```python
from build123d import *

# Parameters (mm, degrees)
SKETCH1_R           = 29.25
SKETCH1_R_2         = 22.025
BOSS_EXTRUDE1_DEPTH = 7
CUT_EXTRUDE1_START  = 7
SKETCH1_3_R         = 1.55
CUT_EXTRUDE1_DEPTH  = 4
SKETCH4_R           = 22.25
SKETCH4_R_2         = 21
BOSS_EXTRUDE2_DEPTH = 1
SKETCH3_R           = 1.55
CUT_EXTRUDE2_DEPTH  = 42.953843686


with BuildPart() as part:
    # Sketch1 → Boss-Extrude1 (new body)
    with BuildSketch(Plane.XY):
        Circle(SKETCH1_R)
        Circle(SKETCH1_R_2, mode=Mode.SUBTRACT)
    extrude(amount=BOSS_EXTRUDE1_DEPTH)

    # Sketch1<3> → Cut-Extrude1 (cut)
    with BuildSketch(Plane.XY.offset(CUT_EXTRUDE1_START)):
        with Locations((0, 25)):
            Circle(SKETCH1_3_R)
        with Locations((10.847093478, 22.524221698)):
            Circle(SKETCH1_3_R)
        with Locations((19.545787062, 15.587245046)):
            Circle(SKETCH1_3_R)
        with Locations((24.373197805, 5.563023349)):
            Circle(SKETCH1_3_R)
        with Locations((24.373197805, -5.563023349)):
            Circle(SKETCH1_3_R)
        with Locations((19.545787062, -15.587245046)):
            Circle(SKETCH1_3_R)
        with Locations((10.847093478, -22.524221698)):
            Circle(SKETCH1_3_R)
        with Locations((0, -25)):
            Circle(SKETCH1_3_R)
        with Locations((-10.847093478, -22.524221698)):
            Circle(SKETCH1_3_R)
        with Locations((-19.545787062, -15.587245046)):
            Circle(SKETCH1_3_R)
        with Locations((-24.373197805, -5.563023349)):
            Circle(SKETCH1_3_R)
        with Locations((-24.373197805, 5.563023349)):
            Circle(SKETCH1_3_R)
        with Locations((-19.545787062, 15.587245046)):
            Circle(SKETCH1_3_R)
        with Locations((-10.847093478, 22.524221698)):
            Circle(SKETCH1_3_R)
    extrude(amount=-CUT_EXTRUDE1_DEPTH, mode=Mode.SUBTRACT)

    # Sketch4 → Boss-Extrude2 (add)
    with BuildSketch(Plane.XY):
        Circle(SKETCH4_R)
        Circle(SKETCH4_R_2, mode=Mode.SUBTRACT)
    extrude(amount=BOSS_EXTRUDE2_DEPTH)

    # Sketch3 → Cut-Extrude2 (cut, through all)
    with BuildSketch(Plane.XY):
        with Locations((5.89680475, 25.835589673)):
            Circle(SKETCH3_R)
        with Locations((23.875674999, 11.497919087)):
            Circle(SKETCH3_R)
        with Locations((23.875674999, -11.497919087)):
            Circle(SKETCH3_R)
        with Locations((5.89680475, -25.835589673)):
            Circle(SKETCH3_R)
        with Locations((-16.522479749, -20.718534285)):
            Circle(SKETCH3_R)
        with Locations((-26.5, 0)):
            Circle(SKETCH3_R)
        with Locations((-16.522479749, 20.718534285)):
            Circle(SKETCH3_R)
    extrude(amount=CUT_EXTRUDE2_DEPTH, mode=Mode.SUBTRACT)


solid = part.part
```
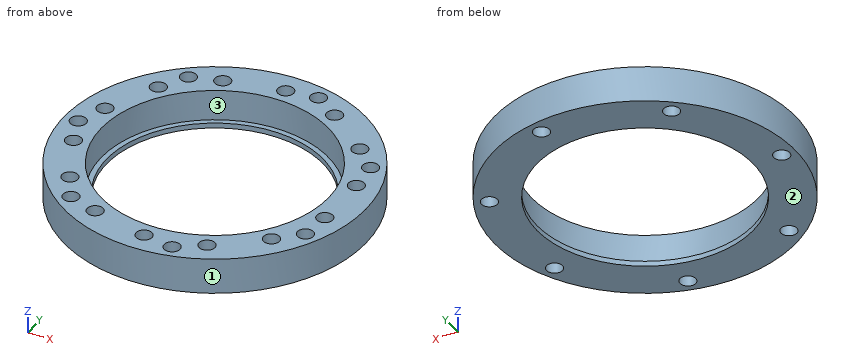
Geometry check sheet. Reference: the model listing, model coordinates, mm. Face numbers are marked on the shaded views. Coordinates: 2 decimals unless noted, no trailing zeros. Write each loop counter-clockwise with the first axis right and the second up, starting at its lowest first coordinate (ties: lowest second). Pieces come first, ordered by that corner, then holes. Notation, with made-up numbers: M 0,-16.75 L 7,-16.75 A25 cw 7,14.25 Z; hole C 69.5,2 d6. An arc over 180 degrees is marked long. One line per item, written item: value. Start each with the question number.
(1) Depth check by flat-ended pin: pin 1 (3.5 mm diameter, centred on x = -16.52, y = -20.72, fed in from -Z); pin 2 (3 mm diameter, centred on x = 0, y = 25, fed in from +Z); pin 3 (4 mm diameter, centred on x = 18.5, z = 6, fed in from +Y); pin 4 (3 mm diameter, centred on x = -23, z = 1, fed in from -Y). Enter the tip coordinate at first touch or a pass-through.
(2) Sectioned sample at D-D, the plane z = 6. State how many separate pieces and enclosed holes the cut face has, and give its area (3 significant figures).
(3) Scan lines: line 1 along X through (y, z) = (-12.5, 6.75); line 2 along Y through (x, z) = (-16.5, 3.75); line 3 along X through (y, z) = (-16, 6.5). Record each from-to range of solid material in increasing order. Write a range as [from, to].
(4) Sectioned sample at C-C, the plane y = -25. Enter the section's corners in (x, z).
(5) Sectioned sample at B-B, the plane x = 0. Enter the section's corners in (y, z) (3 decimals).
(6) Release check for a two-part mould opening along X. For the marked faces 1, 2 and 3 record: released by +X, released by -X, zero draft, split by the parting line, or undercut.
(7) Sectioned sample at A-A, the plane y = 0. Enter the section's corners in (x, z) (3 decimals).
Filled sheet:
1. pin 1: z = 0
1. pin 2: z = 3
1. pin 3: y = 24.15
1. pin 4: y = -19.83
2. separate pieces: 1
2. enclosed holes: 22
2. area: 1,010 mm²
3. line 1: [-26.44, -18.13], [18.13, 22.69], [25.06, 26.44]
3. line 2: [-24.15, -22.27], [-19.17, -14.59], [14.59, 19.17], [22.27, 24.15]
3. line 3: [-24.49, -21.04], [-18.05, -15.14], [15.14, 18.05], [21.04, 24.49]
4. outline: M -15.18,0 L 4.59,0 L 4.59,7 L 1.55,7 L 1.55,3 L -1.55,3 L -1.55,7 L -15.18,7 Z; M 7.2,0 L 15.18,0 L 15.18,7 L 7.2,7 Z
5. outline: M -29.25,0 L -21,0 L -21,1 L -22.025,1 L -22.025,7 L -23.45,7 L -23.45,3 L -26.55,3 L -26.55,7 L -29.25,7 Z; M 21,0 L 29.25,0 L 29.25,7 L 26.55,7 L 26.55,3 L 23.45,3 L 23.45,7 L 22.025,7 L 22.025,1 L 21,1 Z
6. face 1: split by the parting line
6. face 2: zero draft
6. face 3: undercut
7. outline: M -29.25,0 L -28.05,0 L -28.05,7 L -29.25,7 Z; M -24.95,0 L -21,0 L -21,1 L -22.025,1 L -22.025,7 L -24.95,7 Z; M 21,0 L 29.25,0 L 29.25,7 L 22.025,7 L 22.025,1 L 21,1 Z
